```python
from build123d import *

# Parameters (mm, degrees)
ESQUISSE1_W                   = 261.4
ESQUISSE1_H                   = 50
BOSS_EXTRU_1_DEPTH            = 30.2
ENL_V_MAT_EXTRU_3_DEPTH       = 268.846971235
ENL_V_MAT_EXTRU_3_DEPTH_BACK  = 6.2
ENL_V_MAT_EXTRU_4_DEPTH       = 268.846971235
ENL_V_MAT_EXTRU_4_DEPTH_BACK  = 6.2
ENL_V_MAT_EXTRU_6_DEPTH       = 268.846971235
ENL_V_MAT_EXTRU_6_DEPTH_BACK  = 6.2
ENL_V_MAT_EXTRU_7_DEPTH       = 262.799694423
ENL_V_MAT_EXTRU_7_DEPTH_BACK  = 249
ENL_V_MAT_EXTRU_9_DEPTH       = 262.799694423
ENL_V_MAT_EXTRU_9_DEPTH_BACK  = 249
ENL_V_MAT_EXTRU_11_DEPTH      = 268.846971235
ENL_V_MAT_EXTRU_11_DEPTH_BACK = 24
ENL_V_MAT_EXTRU_12_DEPTH      = 268.846971235
ENL_V_MAT_EXTRU_12_DEPTH_BACK = 24
ENL_V_MAT_EXTRU_13_DEPTH      = 268.218936455
ENL_V_MAT_EXTRU_13_DEPTH_BACK = 24
ENL_V_MAT_EXTRU_14_DEPTH      = 268.218936455
ENL_V_MAT_EXTRU_14_DEPTH_BACK = 24
ENL_V_MAT_EXTRU_15_DEPTH      = 268.218936455
ENL_V_MAT_EXTRU_15_DEPTH_BACK = 24
ENL_V_MAT_EXTRU_16_DEPTH      = 268.218936455
ENL_V_MAT_EXTRU_16_DEPTH_BACK = 24
ESQUISSE22_W                  = 220
ESQUISSE22_H                  = 24
BOSS_EXTRU_2_DEPTH            = 10
ESQUISSE23_W                  = 15
ESQUISSE23_H                  = 40
ENL_V_MAT_EXTRU_18_DEPTH      = 24
ESQUISSE24_W                  = 12.5
ESQUISSE24_H                  = 40
ENL_V_MAT_EXTRU_24_DEPTH      = 30
ENL_V_MAT_EXTRU_25_DEPTH      = 270.89257122
ENL_V_MAT_EXTRU_25_DEPTH_BACK = 30
ESQUISSE33_W                  = 30
ESQUISSE33_H                  = 30
ENL_V_MAT_EXTRU_26_DEPTH      = 20
ESQUISSE34_R                  = 2
BOSS_EXTRU_6_DEPTH            = 30
ESQUISSE35_W                  = 30
ESQUISSE35_H                  = 30
ENL_V_MAT_EXTRU_27_DEPTH      = 20
ESQUISSE36_R                  = 2
BOSS_EXTRU_7_DEPTH            = 30


with BuildPart() as part:
    # Esquisse1 → Boss.-Extru.1 (new body)
    with BuildSketch(Plane.XY):
        with Locations((130.7, 25)):
            Rectangle(ESQUISSE1_W, ESQUISSE1_H)
    extrude(amount=BOSS_EXTRU_1_DEPTH)

    # Esquisse2 → Enlèv. mat.-Extru.3 (cut, two sides: drawn at the far end of the back side and taken through both)
    with BuildSketch(Plane.XY.offset(30.2).offset(-ENL_V_MAT_EXTRU_3_DEPTH_BACK)):
        Polygon((797.631736025, 20), (261.4, 20), (0, 20), (-536.231736025, 20), (-536.231736025, 1092.46347205), (797.631736025, 1092.46347205), align=None)
    extrude(amount=ENL_V_MAT_EXTRU_3_DEPTH + ENL_V_MAT_EXTRU_3_DEPTH_BACK, mode=Mode.SUBTRACT)

    # Esquisse5 → Enlèv. mat.-Extru.4 (cut, two sides: drawn at the far end of the back side and taken through both)
    with BuildSketch(Plane.XY.offset(30.2).offset(-ENL_V_MAT_EXTRU_4_DEPTH_BACK)):
        Polygon((6.2, -530.103989602), (6.2, 0), (6.2, 20), (6.2, 550.103989602), (-1054.007979204, 550.103989602), (-1054.007979204, -530.103989602), align=None)
    extrude(amount=ENL_V_MAT_EXTRU_4_DEPTH + ENL_V_MAT_EXTRU_4_DEPTH_BACK, mode=Mode.SUBTRACT)

    # Esquisse6 → Enlèv. mat.-Extru.6 (cut, two sides: drawn at the far end of the back side and taken through both)
    with BuildSketch(Plane.XY.offset(30.2).offset(-ENL_V_MAT_EXTRU_6_DEPTH_BACK)):
        Polygon((255.2, 550.103989602), (255.2, 20), (255.2, 0), (255.2, -530.103989602), (1315.407979204, -530.103989602), (1315.407979204, 550.103989602), align=None)
    extrude(amount=ENL_V_MAT_EXTRU_6_DEPTH + ENL_V_MAT_EXTRU_6_DEPTH_BACK, mode=Mode.SUBTRACT)

    # Esquisse8 → Enlèv. mat.-Extru.7 (cut, two sides: drawn at the far end of the back side and taken through both)
    with BuildSketch(Plane(origin=(255.2, 0, 0), x_dir=(0, 0, -1), z_dir=(1, 0, 0)).offset(-ENL_V_MAT_EXTRU_7_DEPTH_BACK)):
        Polygon((-24, -120.923396991), (-24, 0), (-24, 7.55), (-25.55, 7.55), (-25.55, 3.85), (-26.504639672, 3.85), (-30.2, 7.30657519), (-118.511368381, 89.911479128), (-339.199142385, -9.016667344), (-244.687774004, -219.851543463), align=None)
    extrude(amount=ENL_V_MAT_EXTRU_7_DEPTH + ENL_V_MAT_EXTRU_7_DEPTH_BACK, mode=Mode.SUBTRACT)

    # Esquisse9 → Enlèv. mat.-Extru.9 (cut, two sides: drawn at the far end of the back side and taken through both)
    with BuildSketch(Plane(origin=(255.2, 0, 0), x_dir=(0, 0, -1), z_dir=(1, 0, 0)).offset(-ENL_V_MAT_EXTRU_9_DEPTH_BACK)):
        Polygon((-24, 126.070686284), (-24, 20), (-24, 12.45), (-25.55, 12.45), (-25.55, 16.15), (-26.55, 16.15), (-30.2, 12.645559959), (-106.713439711, -60.816566558), (-300.704336754, 25.040837428), (-217.990897044, 211.92809027), align=None)
    extrude(amount=ENL_V_MAT_EXTRU_9_DEPTH + ENL_V_MAT_EXTRU_9_DEPTH_BACK, mode=Mode.SUBTRACT)

    # Esquisse10 → Enlèv. mat.-Extru.11 (cut, two sides: drawn at the far end of the back side and taken through both)
    with BuildSketch(Plane(origin=(0, 0, 0), x_dir=(-1, 0, 0), z_dir=(0, 0, -1)).offset(-ENL_V_MAT_EXTRU_11_DEPTH_BACK)):
        Polygon((536.231736025, 20), (0, 20), (-20.7, 20), (-20.7, 50), (-20.7, 586.231736025), (743.899228974, 1338.272903737), (1300.830964999, 772.041167712), align=None)
    extrude(amount=ENL_V_MAT_EXTRU_11_DEPTH + ENL_V_MAT_EXTRU_11_DEPTH_BACK, mode=Mode.SUBTRACT)

    # Esquisse11 → Enlèv. mat.-Extru.12 (cut, two sides: drawn at the far end of the back side and taken through both)
    with BuildSketch(Plane(origin=(0, 0, 0), x_dir=(-1, 0, 0), z_dir=(0, 0, -1)).offset(-ENL_V_MAT_EXTRU_12_DEPTH_BACK)):
        Polygon((-797.631736025, 20), (-261.4, 20), (-240.7, 20), (-240.7, 50), (-240.7, 586.231736025), (-1005.299228974, 1338.272903737), (-1562.230964999, 772.041167712), align=None)
    extrude(amount=ENL_V_MAT_EXTRU_12_DEPTH + ENL_V_MAT_EXTRU_12_DEPTH_BACK, mode=Mode.SUBTRACT)

    # Esquisse12 → Enlèv. mat.-Extru.13 (cut, two sides: drawn at the far end of the back side and taken through both)
    with BuildSketch(Plane.XY.offset(24).offset(-ENL_V_MAT_EXTRU_13_DEPTH_BACK)):
        Polygon((6.2, 0), (6.2, 7.55), (4.65, 7.55), (4.65, 3.85), (3.65, 3.85), (0, 7.354440041), (0, 0), align=None)
    extrude(amount=ENL_V_MAT_EXTRU_13_DEPTH + ENL_V_MAT_EXTRU_13_DEPTH_BACK, mode=Mode.SUBTRACT)

    # Esquisse13 → Enlèv. mat.-Extru.14 (cut, two sides: drawn at the far end of the back side and taken through both)
    with BuildSketch(Plane.XY.offset(24).offset(-ENL_V_MAT_EXTRU_14_DEPTH_BACK)):
        Polygon((-388.163092547, -360.037805495), (0, 12.645559959), (3.65, 16.15), (4.65, 16.15), (4.65, 12.45), (6.2, 12.45), (6.2, 20), (6.2, 558.111026928), (-982.664286619, 982.847806423), (-1377.027379166, 64.698974), align=None)
    extrude(amount=ENL_V_MAT_EXTRU_14_DEPTH + ENL_V_MAT_EXTRU_14_DEPTH_BACK, mode=Mode.SUBTRACT)

    # Esquisse16 → Enlèv. mat.-Extru.15 (cut, two sides: drawn at the far end of the back side and taken through both)
    with BuildSketch(Plane.XY.offset(24).offset(-ENL_V_MAT_EXTRU_15_DEPTH_BACK)):
        Polygon((255.2, 20), (255.2, 12.45), (256.75, 12.45), (256.75, 16.15), (257.75, 16.15), (261.4, 12.645559959), (261.4, 20), align=None)
    extrude(amount=ENL_V_MAT_EXTRU_15_DEPTH + ENL_V_MAT_EXTRU_15_DEPTH_BACK, mode=Mode.SUBTRACT)

    # Esquisse17 → Enlèv. mat.-Extru.16 (cut, two sides: drawn at the far end of the back side and taken through both)
    with BuildSketch(Plane.XY.offset(24).offset(-ENL_V_MAT_EXTRU_16_DEPTH_BACK)):
        Polygon((650.717680613, 381.146349234), (261.4, 7.354440041), (257.75, 3.85), (256.75, 3.85), (256.75, 7.55), (255.2, 7.55), (255.2, 0), (255.2, -539.711633945), (1247.009188557, -965.703564334), (1642.52686917, -44.845581155), align=None)
    extrude(amount=ENL_V_MAT_EXTRU_16_DEPTH + ENL_V_MAT_EXTRU_16_DEPTH_BACK, mode=Mode.SUBTRACT)

    # Esquisse22 → Boss.-Extru.2 (add)
    with BuildSketch(Plane(origin=(0, 50, 0), x_dir=(1, 0, 0), z_dir=(0, 1, 0))):
        with Locations((130.7, -12)):
            Rectangle(ESQUISSE22_W, ESQUISSE22_H)
    extrude(amount=BOSS_EXTRU_2_DEPTH)

    # Esquisse23 → Enlèv. mat.-Extru.18 (cut)
    with BuildSketch(Plane(origin=(0, 0, 0), x_dir=(-1, 0, 0), z_dir=(0, 0, -1))):
        with Locations((-233.2, 40)):
            Rectangle(ESQUISSE23_W, ESQUISSE23_H)
    extrude(amount=-ENL_V_MAT_EXTRU_18_DEPTH, mode=Mode.SUBTRACT)

    # Esquisse24 → Enlèv. mat.-Extru.24 (cut)
    with BuildSketch(Plane(origin=(0, 0, 0), x_dir=(-1, 0, 0), z_dir=(0, 0, -1))):
        with Locations((-219.45, 40)):
            Rectangle(ESQUISSE24_W, ESQUISSE24_H)
    extrude(amount=-ENL_V_MAT_EXTRU_24_DEPTH, mode=Mode.SUBTRACT)

    # Esquisse32 → Enlèv. mat.-Extru.25 (cut, two sides: drawn at the far end of the back side and taken through both)
    with BuildSketch(Plane(origin=(0, 0, 0), x_dir=(-1, 0, 0), z_dir=(0, 0, -1)).offset(-ENL_V_MAT_EXTRU_25_DEPTH_BACK)):
        Polygon((477.302008193, 20), (-20.7, 20), (-48.2, 20), (-48.2, 60), (-48.2, 558.002008193), (664.309819102, 1253.957292919), (1189.811827295, 715.955284726), align=None)
    extrude(amount=ENL_V_MAT_EXTRU_25_DEPTH + ENL_V_MAT_EXTRU_25_DEPTH_BACK, mode=Mode.SUBTRACT)

    # Esquisse33 → Enlèv. mat.-Extru.26 (cut)
    with BuildSketch(Plane(origin=(0, 0, 0), x_dir=(-1, 0, 0), z_dir=(0, 0, -1))):
        with Locations((-193.2, 40)):
            Rectangle(ESQUISSE33_W, ESQUISSE33_H)
    extrude(amount=-ENL_V_MAT_EXTRU_26_DEPTH, mode=Mode.SUBTRACT)

    # Esquisse34 → Boss.-Extru.6 (add)
    with BuildSketch(Plane(origin=(0, 0, 20), x_dir=(-1, 0, 0), z_dir=(0, 0, -1))):
        with Locations((-193.2, 40)):
            Circle(ESQUISSE34_R)
    extrude(amount=BOSS_EXTRU_6_DEPTH)

    # Esquisse35 → Enlèv. mat.-Extru.27 (cut)
    with BuildSketch(Plane(origin=(0, 0, 0), x_dir=(-1, 0, 0), z_dir=(0, 0, -1))):
        with Locations((-68.2, 40)):
            Rectangle(ESQUISSE35_W, ESQUISSE35_H)
    extrude(amount=-ENL_V_MAT_EXTRU_27_DEPTH, mode=Mode.SUBTRACT)

    # Esquisse36 → Boss.-Extru.7 (add)
    with BuildSketch(Plane(origin=(0, 0, 20), x_dir=(-1, 0, 0), z_dir=(0, 0, -1))):
        with Locations((-68.2, 40)):
            Circle(ESQUISSE36_R)
    extrude(amount=BOSS_EXTRU_7_DEPTH)


solid = part.part
```
CAD build for the part. Positions are in the model's coordinates, mm. A direction names the side the tool comes from. Give positions to 0.01 mm unless a question says otherwise; leave off trailing zeros. Order: outer loops, then holes, each group sorted by start corner. A loop starts at its lowest first (then second) coordinate and runs counter-clockwise, first axis right, second up. Notation, with made-up numbers: M 48.5,30 L 69.5,30 A16 ccw 69.5,46 Z; hole C 47.5,-4 d6. An arc over 180 degrees is marked long. Put each result on its own line as item: value. Start each with the question number.
(1) Saw through at C-C, the plane x = 38. Write the cut outline in (y, z), then the cut area to 3 significant figures.
(2) Which spindle directions (+Z, -Z, +X, -X, +Y, -Y) get a long thin tool onto all of the face, cutting with end or side? Do faces 4 (the flat face through (3, 10, 24)), 5 (the flat face through (48.2, 40, 12)), 6 (the flat face through (255.2, 10, 27)), 7 (the flat face through (255.2, 16, 12)), 8 (the flat face through (83.2, 40, 10)). Say none if no direction does.
(3) Flat gauge pins, fed straight in: pin 1 Ø1 at (x, z) = (46.5, 9) entering from +Y; pin 2 Ø3 at (y, z) = (46.5, 5) entering from -X; pin 3 Ø1.2 at (x, z) = (5.5, 9) entering from +Y. Where does each tip first touch, or does it go through?
(4) Saw through at D-D, the plane z = 13. Give the number of separate pieces and of enclosed holes in the cut face, then the cut area to 3 significant figures.
(5) Drill centre lines: line 1 along Z through (x, y) = (221, 7.5); line 2 along X through (y, z) = (50, 11.5); line 3 along Z through (x, y) = (187, 28). Where is each one in solid material? Low to high.
(6) Saw through at A-A, the plane y = 48. Write the cut outline in (x, z), then the cut area to 3 significant figures.
(7) Saw through at B-B, the plane z = -6.5. Write the cut outline in (x, y), then the cut area to 3 significant figures.
(8) Mould opens along Y. For faces 1 (the flat face through (130, 60, 12)), 2 (the flat face through (129, 36, 24)), 3 (the flat face through (190, 40, 20)) say: +Y half, -Y half, draft (parallel to the pull), parting line (faces both ways), or undercut.
Check result:
1. outline: M 0,0 L 20,0 L 20,24 L 12.45,24 L 12.45,25.55 L 16.15,25.55 L 16.15,26.55 L 12.65,30.2 L 7.31,30.2 L 3.85,26.5 L 3.85,25.55 L 7.55,25.55 L 7.55,24 L 0,24 Z
1. area: 532 mm2
2. face 4: +Z, -X, +Y, -Y
2. face 5: +Z, -Z, -X, +Y
2. face 6: +Z, +X, +Y, -Y
2. face 7: +Z, -Z, +Y
2. face 8: -Z
3. pin 1: stops at y = 20
3. pin 2: stops at x = 48.2
3. pin 3: stops at y = 12.45
4. separate pieces: 3
4. enclosed holes: 2
4. area: 9,910 mm2
5. line 1: z = 0 to 24, 25.55 to 30.2
5. line 2: x = 48.2 to 53.2, 83.2 to 178.2, 208.2 to 213.2
5. line 3: z = 20 to 24
6. outline: M 48.2,0 L 53.2,0 L 53.2,20 L 83.2,20 L 83.2,0 L 178.2,0 L 178.2,20 L 208.2,20 L 208.2,0 L 213.2,0 L 213.2,24 L 48.2,24 Z
6. area: 2,760 mm2
7. outline: C 68.2,40 d4; C 193.2,40 d4
7. area: 25.1 mm2
8. face 1: +Y half
8. face 2: draft
8. face 3: undercut
